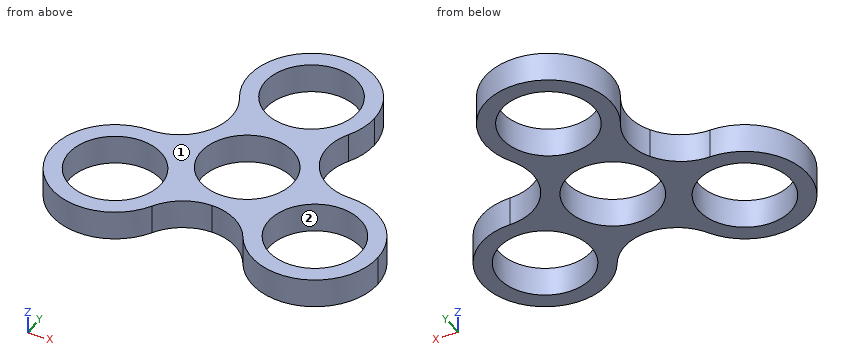
```python
from build123d import *

# Parameters (mm, degrees)
F0_R     = 11
F1_DEPTH = 7
F2_R     = 12.499


# Not quite as in the source:
# - a fillet or chamfer is up to 0.001 mm smaller than in the source, because OpenCascade refuses the exact size


with BuildPart() as f1:
    # F0 (on Top) → F1 (new body)
    with BuildSketch(Plane.XY):
        with BuildLine():
            ThreePointArc((14.9052440041, -1.6833600857), (14.9762922658, -0.8430124372), (15, 0))
            ThreePointArc((15, 0), (12.5483433381, 8.2182163192), (5.9947894041, 13.75))
            ThreePointArc((5.9947894041, 13.75), (0, 12.5), (-5.9947894041, 13.75))
            ThreePointArc((-5.9947894041, 13.75), (-12.9903810568, 7.5), (-14.9052440041, -1.6833600857))
            ThreePointArc((-14.9052440041, -1.6833600857), (-10.8253175473, -6.25), (-8.9104546, -12.0666399143))
            ThreePointArc((-8.9104546, -12.0666399143), (0, -15), (8.9104546, -12.0666399143))
            ThreePointArc((8.9104546, -12.0666399143), (10.8253175473, -6.25), (14.9052440041, -1.6833600857))
        make_face()
        Circle(F0_R, mode=Mode.SUBTRACT)
        with BuildLine():
            ThreePointArc((-5.9947894041, 13.75), (0, 12.5), (5.9947894041, 13.75))
            ThreePointArc((5.9947894041, 13.75), (0, 15), (-5.9947894041, 13.75))
        make_face()
        with BuildLine():
            ThreePointArc((-5.9947894041, 13.75), (0, 15), (5.9947894041, 13.75))
            ThreePointArc((5.9947894041, 13.75), (12.5483433381, 19.2817836808), (15, 27.5))
            ThreePointArc((15, 27.5), (-8.2182163192, 40.0483433381), (-5.9947894041, 13.75))
        make_face()
        with Locations((0, 27.5)):
            Circle(F0_R, mode=Mode.SUBTRACT)
        with BuildLine():
            ThreePointArc((38.8156986041, -13.75), (30.5737745507, -0.3586442247), (14.9052440041, -1.6833600857))
            ThreePointArc((14.9052440041, -1.6833600857), (12.9903810568, -7.5), (8.9104546, -12.0666399143))
            ThreePointArc((8.9104546, -12.0666399143), (22.9726861669, -28.7262922658), (38.8156986041, -13.75))
        make_face()
        with Locations((23.8156986041, -13.75)):
            Circle(F0_R, mode=Mode.SUBTRACT)
        with BuildLine():
            ThreePointArc((8.9104546, -12.0666399143), (12.9903810568, -7.5), (14.9052440041, -1.6833600857))
            ThreePointArc((14.9052440041, -1.6833600857), (10.8253175473, -6.25), (8.9104546, -12.0666399143))
        make_face()
        with BuildLine():
            ThreePointArc((-8.9104546, -12.0666399143), (-10.8253175473, -6.25), (-14.9052440041, -1.6833600857))
            ThreePointArc((-14.9052440041, -1.6833600857), (-12.9903810568, -7.5), (-8.9104546, -12.0666399143))
        make_face()
        with BuildLine():
            ThreePointArc((-8.9104546, -12.0666399143), (-12.9903810568, -7.5), (-14.9052440041, -1.6833600857))
            ThreePointArc((-14.9052440041, -1.6833600857), (-37.2070543793, -20.5080759466), (-8.8156986041, -13.75))
            ThreePointArc((-8.8156986041, -13.75), (-8.8394063383, -12.9069875628), (-8.9104546, -12.0666399143))
        make_face()
        with Locations((-23.8156986041, -13.75)):
            Circle(F0_R, mode=Mode.SUBTRACT)
    extrude(amount=F1_DEPTH)

    # F2 (radius 12.5 in the source; OpenCascade refuses exactly that, so slightly less here)
    f2_edges = [f1.edges().sort_by_distance(p)[0] for p in [
        (-5.994789, 13.75, 3.5),
        (14.905244, -1.68336, 3.5),
        (-14.905244, -1.68336, 3.5),
        (5.994789, 13.75, 3.5),
        (-8.910455, -12.06664, 3.5),
        (8.910455, -12.06664, 3.5),
    ]]
    fillet(f2_edges, radius=F2_R)


solid = f1.part
```
Read the model definition and answer for the solid it produces. Units are mm, in the model's axes. Face numbers are marked on the shaded views. Coordinates: 2 decimals unless noted, no trailing zeros. Write each loop counter-clockwise with the first axis right and the second up, starting at its lowest first coordinate (ties: lowest second). Pieces come first, ordered by that corner, then holes. Notation, with made-up numbers: (47, 58.5) - (84, 58.5) arc R20 cw to (84, 64.5) - close; hole circle Ø9 at (48.25, 61.5). An arc over 180 degrees is marked (long way). Answer as a JSON object with one key per item and string values. Group by question number.
1. A cutting plane is placed at A-A (y = -10). Determine the outline of the cut face in (x, z).
2. Each of these flat-tipped pins is pushed along its axis until it touches: P1, Ø4, axis at x = -29.5, z = 5.5, coming from the -Y side; P2, Ø3, axis at x = 29.5, z = 5, coming from the +Y side; P3, Ø1, axis at x = -4, z = 6, coming from the +Y side. Where does it stop, or does it pass through?
3. Consider L1, parallel to Y at x = 0, z = 4.5; L2, parallel to Y at x = 4, z = 3.5; L3, parallel to X at y = -21, z = 5.25. Determine where each line is inside the solid, lowest interval first. Write a range as [from, to].
4. A cutting plane is placed at B-B (x = 33.5). Determine the outline of the cut face in (y, z), plus the area to 3 significant figures.
5. The mould has two halves that part along X. Classify the marked faces 1 and 2: +X half, -X half, draft (parallel to the pull), parting line (faces both ways), or undercut.
6. A cutting plane is placed at C-C (y = 0). Determine the outline of the cut face in (x, z).
7. A cutting plane is placed at D-D (z = 4). Give the number of separate pieces and of enclosed holes in the cut face, plus the area to 3 significant figures.
Worked out:
{
 "1": {"outline": "(-38.34, 0) - (-34.16, 0) - (-34.16, 7) - (-38.34, 7) - close; (-13.47, 0) - (-4.58, 0) - (-4.58, 7) - (-13.47, 7) - close; (4.58, 0) - (13.47, 0) - (13.47, 7) - (4.58, 7) - close; (34.16, 0) - (38.34, 0) - (38.34, 7) - (34.16, 7) - close"},
 "2": {"P1": "stops at y = -28.29", "P2": "stops at y = 0.65", "P3": "stops at y = 42.09"},
 "3": {"L1": "y = [-15, -11], [11, 16.5], [38.5, 42.5]", "L2": "y = [-15.66, -10.25], [10.25, 17.25], [37.75, 41.96]", "L3": "x = [-36.95, -32.09], [-15.54, -10.68], [10.68, 15.54], [32.09, 36.95]"},
 "4": {"outline": "(-25.2, 0) - (-18.97, 0) - (-18.97, 7) - (-25.2, 7) - close; (-8.53, 0) - (-2.3, 0) - (-2.3, 7) - (-8.53, 7) - close", "area": "87.3 mm²"},
 "5": {"face 1": "draft", "face 2": "undercut"},
 "6": {"outline": "(-29.81, 0) - (-11, 0) - (-11, 7) - (-29.81, 7) - close; (11, 0) - (29.81, 0) - (29.81, 7) - (11, 7) - close"},
 "7": {"separate pieces": "1", "enclosed holes": "4", "area": "1,370 mm²"}
}
